Geometry: final body of the model. Coordinates: model frame, mm. A direction names the side the tool comes from. Round coordinates to 2 decimals unless told otherwise and drop trailing zeros. Loops run counter-clockwise (first coordinate to the right, second up) from the corner with the lowest first, then second, coordinate; pieces in that order, holes last. Notation, with made-up numbers: M 76.25,28 L 130.25,28 A27 cw 130.25,56 Z; hole C 25,8 d6. An arc over 180 degrees is marked long. Write each question's results on one line, items separated by ' | '.
```python
from build123d import *

# Parameters (mm, degrees)
F0_W     = 55
F0_H     = 19
F1_DEPTH = 11
F2_W     = 18.1
F2_H     = 10.1
F3_DEPTH = 11
F5_DEPTH = 4.5
F7_DEPTH = 4.5
F8_W     = 15.25
F8_H     = 3.25
F9_DEPTH = 52


with BuildPart() as f1:
    # F0 (on Front) → F1 (new body, symmetric)
    with BuildSketch(Plane.XZ):
        Rectangle(F0_W, F0_H)
    extrude(amount=F1_DEPTH, both=True)

    # F2 (on Top) → F3 (cut, symmetric)
    with BuildSketch(Plane.XY):
        with Locations((5, 0)):
            Rectangle(F2_W, F2_H)
    extrude(amount=F3_DEPTH, both=True, mode=Mode.SUBTRACT)

    # F4 (on face) → F5 (cut)
    with BuildSketch(Plane.XZ.offset(-5.05)):
        with BuildLine():
            Line((10.4, 1), (-0.4, 1))
            ThreePointArc((-0.4, 1), (-1.4, 0), (-0.4, -1))
            Line((-0.4, -1), (10.4, -1))
            ThreePointArc((10.4, -1), (11.4, 0), (10.4, 1))
        make_face()
    extrude(amount=-F5_DEPTH, mode=Mode.SUBTRACT)

    # F6 (on face) → F7 (cut)
    with BuildSketch(Plane(origin=(0, -5.05, 0), x_dir=(-1, 0, 0), z_dir=(0, 1, 0))):
        with BuildLine():
            ThreePointArc((-10.4, 1), (-11.4, 0), (-10.4, -1))
            Line((-10.4, -1), (0.4, -1))
            ThreePointArc((0.4, -1), (1.4, 0), (0.4, 1))
            Line((0.4, 1), (-10.4, 1))
        make_face()
    extrude(amount=-F7_DEPTH, mode=Mode.SUBTRACT)

    # F8 (on face) → F9 (cut)
    with BuildSketch(Plane(origin=(-27.5, 0, 0), x_dir=(0, -1, 0), z_dir=(-1, 0, 0))):
        Rectangle(F8_W, F8_H)
    extrude(amount=-F9_DEPTH, mode=Mode.SUBTRACT)


solid = f1.part
```
1. Section B-B (y = -9). Output: boundary loops of the cut face in (x, z), then the cut area to 3 significant figures.
Answer key:
outline: M -27.5,-9.5 L 27.5,-9.5 L 27.5,9.5 L -27.5,9.5 Z; hole M -0.4,-1 L 10.4,-1 A1 ccw 10.4,1 L -0.4,1 A1 ccw Z | area: 1,020 mm²
2. Access query for faces 4 (the face through (11.4, 8.6, 0)), 5 (the face through (5, 5.05, -6)), 6 (the face through (24.5, 0, 0)). Directions: +Z, -Z, +X, -X, +Y, -Y. A direction counts if a zero-diameter tool reaches every point of the face in a straight line with its end or side. Return the directions, or none.
Answer key:
face 4: none | face 5: +Z, -Z | face 6: -X
3. Section C-C (x = -12.5). Output: boundary loops of the cut face in (y, z) (3 decimals).
Answer key:
outline: M -11,-9.5 L 11,-9.5 L 11,9.5 L -11,9.5 Z; hole M -7.625,-1.625 L 7.625,-1.625 L 7.625,1.625 L -7.625,1.625 Z
4. Draft query along Y for faces 1 (the face through (-6, 0, 9.5)), 2 (the face through (0, -11, 0)), 3 (the face through (-4.05, 0, 6)). Return one class per face: pulls with the +Y half, pulls with the -Y half, needs draft (parallel to the pull), parting line crosses it, or undercut.
Answer key:
face 1: needs draft | face 2: pulls with the -Y half | face 3: undercut
5. Ray query, probe 1 along Z at (x, y) = (-8, 6.5) (3 decimals); probe 2 along Y at (x, z) = (14, -5); probe 3 along X at (y, z) = (-0.5, -2.75). Return the intervals inside material, ascending.
Answer key:
probe 1: z = -9.5 to -1.625, 1.625 to 9.5 | probe 2: y = -11 to -5.05, 5.05 to 11 | probe 3: x = -27.5 to -4.05, 14.05 to 27.5
6. Section D-D (z = 0). Output: boundary loops of the cut face in (x, y) (3 decimals), then the cut area to 3 significant figures.
Answer key:
outline: M -27.5,-11 L 27.5,-11 L 27.5,11 L -27.5,11 L -27.5,7.625 L -1.4,7.625 L -1.4,9.55 L 11.4,9.55 L 11.4,7.625 L 24.5,7.625 L 24.5,-7.625 L 11.4,-7.625 L 11.4,-9.55 L -1.4,-9.55 L -1.4,-7.625 L -27.5,-7.625 Z | area: 368 mm²
7. Section A-A (y = 2). Output: boundary loops of the cut face in (x, z) (3 decimals).
Answer key:
outline: M -27.5,-9.5 L -4.05,-9.5 L -4.05,-1.625 L -27.5,-1.625 Z; M -27.5,1.625 L -4.05,1.625 L -4.05,9.5 L -27.5,9.5 Z; M 14.05,-9.5 L 27.5,-9.5 L 27.5,9.5 L 14.05,9.5 L 14.05,1.625 L 24.5,1.625 L 24.5,-1.625 L 14.05,-1.625 Z
8. Pin query (flat end, axial travel): P1, Ø8, axis at x = 4.5, y = 3, coming from the +Z side. Return the tip coordinate at first contact, or that it passes through.
Answer key:
P1: stops at z = 9.5
